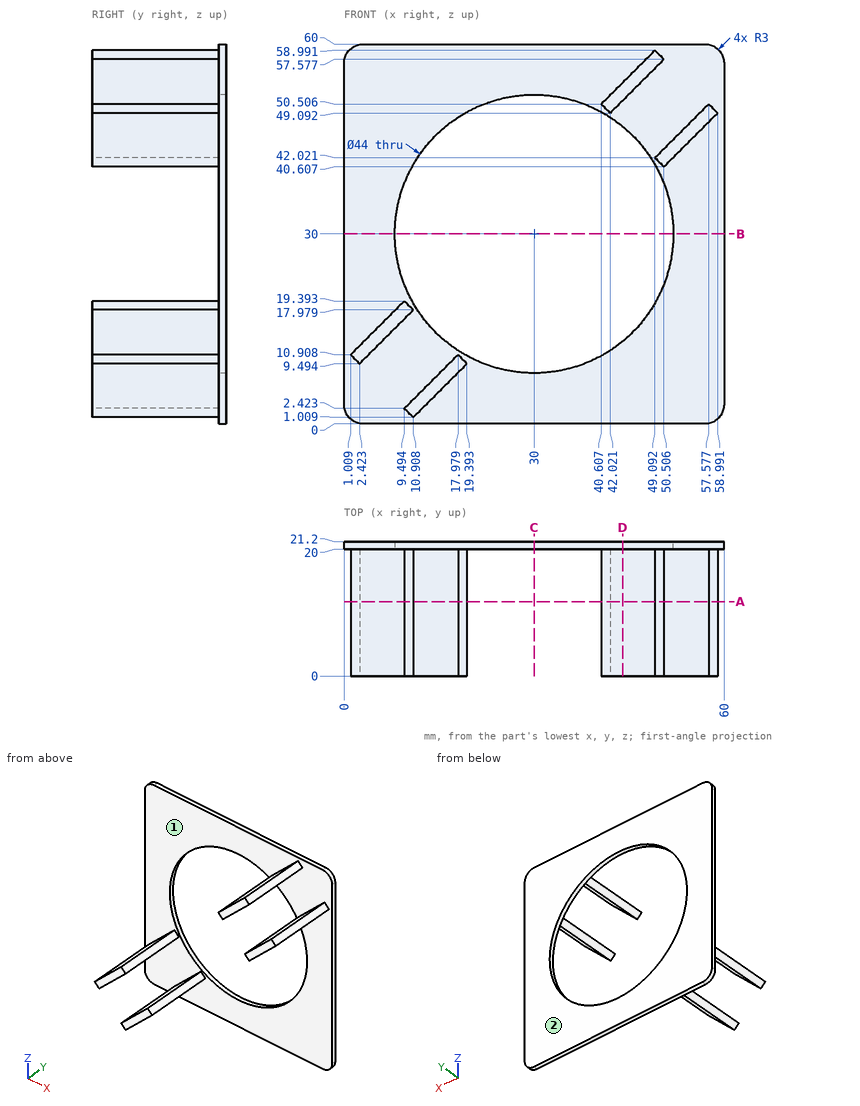
Check sheet for the drawn part. Datum: minimum x, y, z corner. Units: mm. A direction names the side the tool comes from. Round coordinates to 2 decimals unless told otherwise and drop trailing zeros. Order: outer loops, then holes, each group sorted by start corner. A loop starts at its lowest first (then second) coordinate and runs counter-clockwise, first axis right, second up.
(1) Cross-section at D-D, the plane x = 44. Enter the section's corners in (y, z).
(2) Access from +Z, -Z, +X, -X, +Y, -Y to the whole of each face (thin tool, end or side, straight path). Record for the marked faces 1 and 2.
(3) Cross-section at C-C, the plane x = 30. Enter the section's corners in (y, z).
(4) Scan lines: probe 1 along Z at (x, y) = (30, 20.85); probe 2 along Y at (x, z) = (42, 8.5). Record each from-to range of solid material in increasing order.
(5) Cross-section at A-A, the plane y = 11.75. Enter the section's corners in (x, z).
(6) Cross-section at B-B, the plane z = 30. Enter the section's corners in (x, y), and give its area (3 significant figures).
(7) Go/stop test with flat-tipped pins: P1, Ø10, axis at y = 3, z = 7.5, coming from the +X side; P2, Ø6, axis at y = 14.5, z = 38, coming from the -X side; P3, Ø3, axis at x = 9.5, z = 13, coming from the -Y side. Record where each tip stops, or that it passes through.
Check sheet entries:
1. outline: (0, 51.07) - (20, 51.07) - (20, 46.97) - (21.2, 46.97) - (21.2, 60) - (20, 60) - (20, 53.9) - (0, 53.9) - close; (20, 0) - (21.2, 0) - (21.2, 13.03) - (20, 13.03) - close
2. face 1: -Y
2. face 2: +Z, -Z, +X, -X, +Y
3. outline: (20, 0) - (21.2, 0) - (21.2, 8) - (20, 8) - close; (20, 52) - (21.2, 52) - (21.2, 60) - (20, 60) - close
4. probe 1: z = 0 to 8, 52 to 60
4. probe 2: y = 20 to 21.2
5. outline: (1.01, 10.91) - (2.42, 9.49) - (10.91, 17.98) - (9.49, 19.39) - close; (9.49, 2.42) - (10.91, 1.01) - (19.39, 9.49) - (17.98, 10.91) - close; (40.61, 50.51) - (42.02, 49.09) - (50.51, 57.58) - (49.09, 58.99) - close; (49.09, 42.02) - (50.51, 40.61) - (58.99, 49.09) - (57.58, 50.51) - close
6. outline: (0, 20) - (8, 20) - (8, 21.2) - (0, 21.2) - close; (52, 20) - (60, 20) - (60, 21.2) - (52, 21.2) - close
6. area: 19.2 mm2
7. P1: stops at x = 19.39
7. P2: stops at x = 50.11
7. P3: stops at y = 20
